Autodesk Inventor part; units mm, degrees
ref_plane "YZ Plane" through (0, 0, 0) normal (1, 0, 0) x (0, 1, 0)
ref_plane "XZ Plane" through (0, 0, 0) normal (0, 1, 0) x (-1, 0, 0)
ref_plane "XY Plane" through (0, 0, 0) normal (0, 0, 1) x (1, 0, 0)
sketch "Sketch1" plane through (0, 0, 0) normal (0, 1, 0) x (-1, 0, 0)
  line L0 (0, 0) -> (20, 0)
  line L1 (20, 0) -> (20, -82)
  line L2 (20, -82) -> (0, -82)
  line L3 (0, -82) -> (0, 0)
  line L4 (0, 0) -> (-10, 0)
  line L5 (-10, 0) -> (-10, -22)
  line L6 (-10, -22) -> (0, -22)
  line L7 (0, -22) -> (0, 0)
  point P0 (0, -22)
  dimension "d0" = 20
  dimension "d1" = 82
  dimension "d12" = 22
  dimension "d13" = 10
extrude "Extrusion1" add sketch "Sketch1" along normal blind 5
fillet "Fillet1" radius 5 6 edges at (0, 2.5, -82) (-20, 2.5, -82) (-20, 2.5, 0) (10, 2.5, 0) (0, 2.5, -22) (10, 2.5, -22)
sketch "Sketch3" plane through (0, 5, 0) normal (0, 1, 0) x (1, 0, 0)
  line L0 (-24.763, 10) -> (25.9614, 10)
  line L1 (-15, 0) -> (5, 0)
  circle A0 centre (-9, 10) radius 2
  circle A1 centre (-1, 10) radius 2
  line L2 (-20, 77) -> (-20, 5)
  point P0 (0, 0)
  dimension "d14" = 10
  dimension "d15" = 4
  dimension "d16" = 4
  dimension "d17" = 8
  dimension "d18" = 11
hole "Hole2" at (-9, 5, -10) at (-1, 5, -10) direction (0, -1, 0) diameter 4 end through all
sketch "Sketch4" plane through (0, 5, 0) normal (0, 1, 0) x (1, 0, 0)
  circle A0 centre (-10, 64.5) radius 1.5
  circle A1 centre (-10, 39.5) radius 1.5
  point P0 (0, 0)
hole "Hole3" at (-10, 5, -64.5) at (-10, 5, -39.5) direction (0, -1, 0) diameter 3.5 end through all
equation "\"d16\" = d15"
equation "\"d19\" = d15"
properties part number "X-Kettenhalter2"
Design review of the part built by this model. Coordinates are the model's own, in mm. A direction names the side the tool comes from. Give positions to 0.01 mm unless a question says otherwise; leave off trailing zeros. Loops run counter-clockwise (first coordinate to the right, second up) from the corner with the lowest first, then second, coordinate; pieces in that order, holes last. Notation, with made-up numbers: M 23,76.5 L 54,76.5 A33 cw 54,105.5 Z; hole C -6,-12.75 d9. An arc over 180 degrees is marked long. Return JSON: item names as keys, results as strings. Group by question number.
Item 1: Insertion check: pin 1 Ø3 at (y, z) = (1.5, -52) entering from +X. The pin has a flat end and moves straight along its axis. Give the tip position at first contact, or say it passes through.
Item 2: We need section D-D (z = -64.5). Give the boundary of the cut face in (x, y).
Item 3: We need section A-A (z = -10). Give the boundary of the cut face in (x, y), and give its area (3 significant figures).
Item 4: Mouldability with a two-part tool opening along X and no side actions: class faces 3 (the flat face through (-20, 2, -40)), 4 (the cylindrical face through (-11, 2, -10)), 5 (the cylindrical face through (1, 3, -24)), 6 (the cylindrical face through (0.2, 2.5, -11.6)) as released by +X, released by -X, zero draft, split by the parting line, or undercut.
Item 5: We need section B-B (y = 2.4). Give the number of separate pieces and of enclosed holes in the cut face, and give its area (3 significant figures).
Item 6: We need section C-C (x = -10). Give the boundary of the cut face in (y, z).
Item 7: For probe 1 along Z at (x, y) = (-10, 2.5); probe 2 along X at (y, z) = (1.95, -10); probe 3 along X at (y, z) = (2.4, -64.5), list the stretches that pass through material, from the lowest coordinate up.
Item 8: Tool access review of faces 1 (the flat face through (0, 2, -52)), 2 (the flat face through (-8, 0, -40)): name each direction out of +Z, -Z, +X, -X, +Y, -Y from which nothing blocks a thin tool from reaching the whole face with its end or side.
Output:
{
 "1": {"pin 1": "stops at x = 0"},
 "2": {"outline": "M -20,0 L -11.75,0 L -11.75,5 L -20,5 Z; M -8.25,0 L 0,0 L 0,5 L -8.25,5 Z"},
 "3": {"outline": "M -20,0 L -11,0 L -11,5 L -20,5 Z; M -7,0 L -3,0 L -3,5 L -7,5 Z; M 1,0 L 10,0 L 10,5 L 1,5 Z", "area": "110 mm^2"},
 "4": {"face 3": "released by -X", "face 4": "undercut", "face 5": "released by +X", "face 6": "undercut"},
 "5": {"separate pieces": "1", "enclosed holes": "4", "area": "1,790 mm^2"},
 "6": {"outline": "M 0,-82 L 5,-82 L 5,-66.25 L 0,-66.25 Z; M 0,-62.75 L 5,-62.75 L 5,-41.25 L 0,-41.25 Z; M 0,-37.75 L 5,-37.75 L 5,-11.73 L 0,-11.73 Z; M 0,-8.27 L 5,-8.27 L 5,0 L 0,0 Z"},
 "7": {"probe 1": "z = -82 to -66.25, -62.75 to -41.25, -37.75 to -11.73, -8.27 to 0", "probe 2": "x = -20 to -11, -7 to -3, 1 to 10", "probe 3": "x = -20 to -11.75, -8.25 to 0"},
 "8": {"face 1": "-Z, +X, +Y, -Y", "face 2": "+Z, -Z, +X, -X, -Y"}
}
